The drawing under review shows one solid part. Ordinate dimensions are in mm from its lowest x, y, z. Give positions to 0.01 mm unless a question says otherwise; leave off trailing zeros. Order: outer loops, then holes, each group sorted by start corner. A loop starts at its lowest first (then second) coordinate and runs counter-clockwise, first axis right, second up. Notation, with made-up numbers: (40.5, 42) - (45.5, 42) arc R27 ccw to (45.5, 69) - close; hole circle Ø5 at (60, 10.25). An arc over 180 degrees is marked (long way). Use CSV: the item, a comma, the result in double quotes.
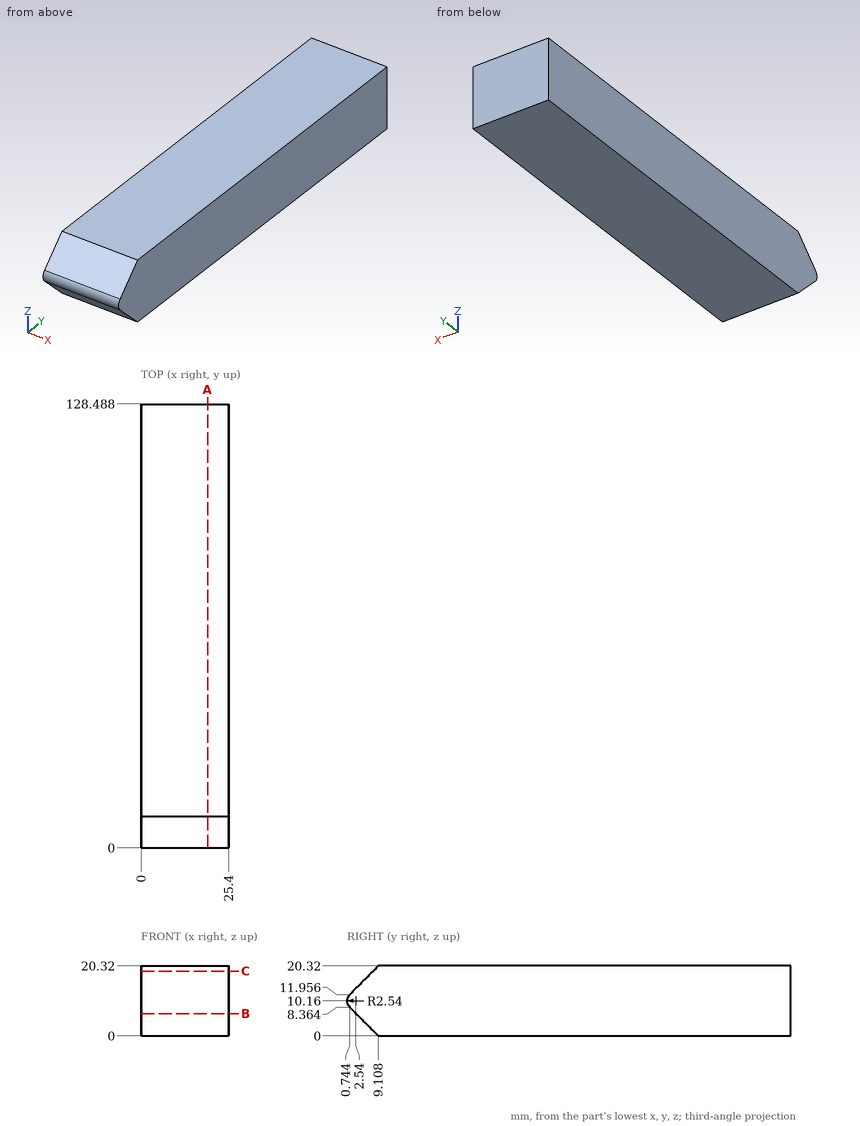
Item 1: Take a section at B-B, the plane z = 6.5. Give the boundary of the cut face in (x, y).
Results list:
outline,"(0, 2.61) - (25.4, 2.61) - (25.4, 128.49) - (0, 128.49) - close"
Item 2: Clearance check with a flat-ended pin moving along its axis: pin 1 (4 mm diameter, centred on x = 3, z = 3.5, fed in from -Y). State where the tip first meets the part, or that it passes through.
Results list:
pin 1,"stops at y = 3.61"
Item 3: Wall thickness on L1, parallel to Y at x = 20.25, z = 10.25; L2, parallel to Y at x = 2.5, z = 11: over which ranges is each line inside the solid? List them lowest first.
Results list:
L1,"y = 0 to 128.49"
L2,"y = 0.14 to 128.49"
Item 4: Take a section at C-C, the plane z = 18.75. Give the boundary of the cut face in (x, y), and give its area (3 significant figures).
Results list:
outline,"(0, 7.54) - (25.4, 7.54) - (25.4, 128.49) - (0, 128.49) - close"
area,"3,070 mm2"
Item 5: Take a section at A-A, the plane x = 19.25. Give the boundary of the cut face in (y, z).
Results list:
outline,"(0.74, 8.36) - (9.11, 0) - (128.49, 0) - (128.49, 20.32) - (9.11, 20.32) - (0.74, 11.96) arc R2.54 ccw to start"
